Autodesk Inventor part; units mm, degrees
ref_plane "YZ Plane" through (0, 0, 0) normal (1, 0, 0) x (0, 1, 0)
ref_plane "XZ Plane" through (0, 0, 0) normal (0, 1, 0) x (-1, 0, 0)
ref_plane "XY Plane" through (0, 0, 0) normal (0, 0, 1) x (1, 0, 0)
sketch "Sketch1" plane through (0, 0, 0) normal (0, 0, 1) x (1, 0, 0)
  line L0 (-68.58, -128.7145) -> (68.58, -128.7145)
  line L1 (68.58, -128.7145) -> (68.58, 128.7145)
  line L2 (68.58, 128.7145) -> (-68.58, 128.7145)
  line L3 (-68.58, 128.7145) -> (-68.58, -128.7145)
  line L4 (-68.58, -128.7145) -> (68.58, 128.7145) construction
  line L5 (68.58, -128.7145) -> (-68.58, 128.7145) construction
  point P0 (0, 0)
  dimension "d0" = 137.16
  dimension "d1" = 257.429
extrude "Extrusion1" add sketch "Sketch1" against normal blind 1.5875
sketch "Sketch2" plane through (0, 0, 0) normal (0, 0, 1) x (1, 0, 0)
  circle A0 centre (-59.69, 52.5145) radius 2.0955
  line L0 (-68.58, 128.7145) -> (-68.58, -128.7145)
  line L1 (-68.58, 128.7145) -> (68.58, 128.7145)
  circle A1 centre (59.69, 52.5145) radius 2.0955
  line L2 (68.58, -128.7145) -> (68.58, 128.7145)
  circle A2 centre (-59.69, -116.0145) radius 2.0955
  circle A3 centre (59.69, -116.0145) radius 2.0955
  line L3 (-68.58, -128.7145) -> (68.58, -128.7145)
  point P0 (0, 0)
  dimension "d4" = 8.89
  dimension "d5" = 76.2
  dimension "d6" = 76.2
  dimension "d7" = 8.89
  dimension "d8" = 4.191
  dimension "d9" = 12.7
  dimension "d10" = 8.89
  dimension "d11" = 8.89
  dimension "d12" = 12.7
  dimension "d13" = 4.191
  dimension "d21" = 4.191
  dimension "d22" = 4.191
hole "Hole1" at (-59.69, 52.5145, 0) at (59.69, 52.5145, 0) at (-59.69, -116.0145, 0) at (59.69, -116.0145, 0) direction (0, 0, -1) diameter 4.191 end through all
sketch "Sketch4" plane through (0, 0, 0) normal (0, 0, 1) x (1, 0, 0)
  line L0 (-35.179, -49.0855) -> (-35.179, -99.8855)
  line L1 (-28.321, -49.0855) -> (-28.321, -99.8855)
  line L2 (28.321, -49.0855) -> (28.321, -99.8855)
  line L3 (35.179, -49.0855) -> (35.179, -99.8855)
  line L4 (-68.58, 128.7145) -> (-68.58, -128.7145)
  line L5 (68.58, -128.7145) -> (68.58, 128.7145)
  line L6 (-68.58, -128.7145) -> (68.58, -128.7145)
  arc A0 (-28.321, -49.0855) -> (-35.179, -49.0855) centre (-31.75, -49.0855) ccw
  arc A1 (-35.179, -99.8855) -> (-28.321, -99.8855) centre (-31.75, -99.8855) ccw
  arc A2 (35.179, -49.0855) -> (28.321, -49.0855) centre (31.75, -49.0855) ccw
  arc A3 (28.321, -99.8855) -> (35.179, -99.8855) centre (31.75, -99.8855) ccw
  point P0 (0, 0)
  dimension "d23" = 6.858
  dimension "d24" = 6.858
  dimension "d25" = 33.401
  dimension "d26" = 50.8
  dimension "d27" = 33.401
  dimension "d28" = 28.829
  dimension "d29" = 28.829
  dimension "d30" = 28.829
  dimension "d31" = 28.829
  dimension "d32" = 50.8
  dimension "d33" = 50.8
  dimension "d34" = 50.8
extrude "Extrusion2" cut sketch "Sketch4" against normal blind 3.175
sketch "Sketch5" plane through (0, 0, 0) normal (0, 0, 1) x (1, 0, 0)
  line L0 (-68.58, 128.7145) -> (68.58, 128.7145)
  line L1 (68.58, 128.7145) -> (68.58, -128.7145)
  point P0 (0, 0)
  point P1 (-43.3324, 96.9645)
  point P2 (43.3324, 96.9645)
  dimension "d37" = 31.75
  dimension "d38" = 86.6648
  dimension "d39" = 31.75
  dimension "d40" = 25.2476
hole "Hole2" at (-43.3324, 96.9645, 0) at (43.3324, 96.9645, 0) direction (0, 0, -1) diameter 4.4704 end through all
sketch "battery_buzzer" plane through (0, 0, 0) normal (0, 0, 1) x (1, 0, 0)
  point P0 (0, 0)
sketch "Sketch10" plane through (0, 0, 0) normal (0, 0, 1) x (1, 0, 0)
  line L0 (-50.8, -128.7145) -> (-50.8, 39.8145)
  line L1 (-50.8, 39.8145) -> (50.8, 39.8145)
  line L2 (50.8, 39.8145) -> (50.8, -128.7145)
  line L3 (68.58, 128.7145) -> (-68.58, 128.7145)
  line L4 (-68.58, 128.7145) -> (-68.58, -128.7145)
  line L5 (68.58, 128.7145) -> (68.58, -128.7145)
  line L6 (-50.8, -128.7145) -> (50.8, -128.7145)
  point P0 (0, 0)
  dimension "d48" = 88.9
  dimension "d49" = 17.78
  dimension "d50" = 17.78
extrude "Extrusion3" cut sketch "Sketch10" against normal blind 3.175
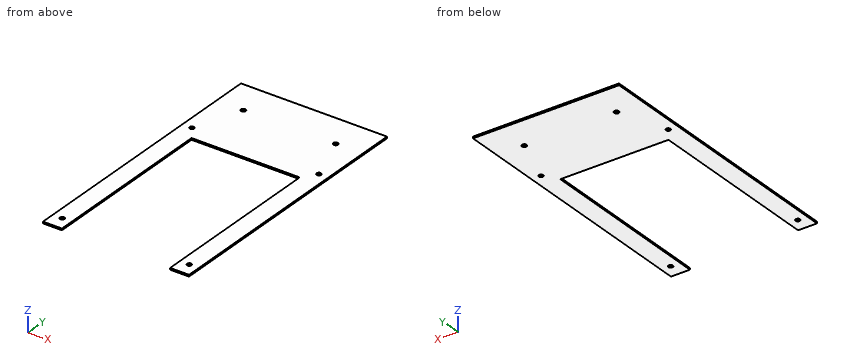
Part model, mm, in its own coordinate system. Round coordinates to 2 decimals unless told otherwise and drop trailing zeros. Loops run counter-clockwise (first coordinate to the right, second up) from the corner with the lowest first, then second, coordinate; pieces in that order, holes last.
1. Slice it at B-B (z = -1.15). Give the cut face in (x, y), and give its area (3 significant figures).
Solutions:
outline: (-68.58, -128.71) - (-50.8, -128.71) - (-50.8, 39.81) - (50.8, 39.81) - (50.8, -128.71) - (68.58, -128.71) - (68.58, 128.71) - (-68.58, 128.71) - close; hole circle Ø4.19 at (-59.69, -116.01); hole circle Ø4.19 at (-59.69, 52.51); hole circle Ø4.47 at (-43.33, 96.96); hole circle Ø4.47 at (43.33, 96.96); hole circle Ø4.19 at (59.69, -116.01); hole circle Ø4.19 at (59.69, 52.51)
area: 18,100 mm2
2. Slice it at C-C (x = -26.5). Give the cut face in (y, z).
Solutions:
outline: (39.81, -1.59) - (128.71, -1.59) - (128.71, 0) - (39.81, 0) - close
3. Drill centre lines: line 1 along Y through (x, z) = (-59.69, -0.3); line 2 along X through (y, z) = (-94.5, -0.7); line 3 along Y through (x, z) = (-14.5, -1.05). Where is each one in solid material? Low to high.
Solutions:
line 1: y = -128.71 to -118.11, -113.92 to 50.42, 54.61 to 128.71
line 2: x = -68.58 to -50.8, 50.8 to 68.58
line 3: y = 39.81 to 128.71
4. Flat gauge pin, fed straight in: pin 1 (5.5 mm diameter, centred on x = 59.69, y = 52.51, fed in from +Z). Where does the tip first touch, or does it go through?
Solutions:
pin 1: stops at z = 0
5. Slice it at A-A (y = -77). Give the cut face in (x, z).
Solutions:
outline: (-68.58, -1.59) - (-50.8, -1.59) - (-50.8, 0) - (-68.58, 0) - close; (50.8, -1.59) - (68.58, -1.59) - (68.58, 0) - (50.8, 0) - close
